The model under review builds one solid part; all positions refer to its coordinate system, in mm. A direction names the side the tool comes from. Coordinates: 2 decimals unless noted, no trailing zeros. Order: outer loops, then holes, each group sorted by start corner. A loop starts at its lowest first (then second) coordinate and runs counter-clockwise, first axis right, second up.
Autodesk Inventor part; units mm, degrees
ref_plane "YZ Plane" through (0, 0, 0) normal (1, 0, 0) x (0, 1, 0)
ref_plane "XZ Plane" through (0, 0, 0) normal (0, 1, 0) x (-1, 0, 0)
ref_plane "XY Plane" through (0, 0, 0) normal (0, 0, 1) x (1, 0, 0)
sketch "Sketch1" plane through (0, 0, 0) normal (0, 1, 0) x (-1, 0, 0)
  circle A0 centre (0, 0) radius 7.5
  dimension "d8" = 15
extrude "Extrusion1" add sketch "Sketch1" along normal blind 53
sketch "Sketch2" plane through (0, 0, 0) normal (0, -1, 0) x (1, 0, 0)
  circle A0 centre (0, 0) radius 1.5
  dimension "d3" = 3
extrude "Extrusion2" add sketch "Sketch2" along normal blind 2
fillet "Fillet1" [suppressed]
fillet "Fillet2" radius 0.4 2 edges at (-1.5, -2, 0) (-1.5, 0, 0)
fillet "Fillet3" radius 1 2 edges at (7.5, 53, 0) (7.5, 0, 0)
properties part number "Battery"
(1) Machinability: for faces 1 (the face through (0, -2, 0)), 2 (the face through (-1, 0, 2)), which of the approach directions +Z, -Z, +X, -X, +Y, -Y give a long, thin tool a straight path to every point of the face, cutting with its end or side? Answer none if there is none.
A:
face 1: +Z, -Z, +X, -X, -Y
face 2: -Y
(2) We need section B-B, the plane z = 0. Write out the cut boundary in (x, y).
A:
outline: (-7.5, 1) arc R1 ccw to (-6.5, 0) - (-1.9, 0) arc R0.4 cw to (-1.5, -0.4) - (-1.5, -1.6) arc R0.4 ccw to (-1.1, -2) - (1.1, -2) arc R0.4 ccw to (1.5, -1.6) - (1.5, -0.4) arc R0.4 cw to (1.9, 0) - (6.5, 0) arc R1 ccw to (7.5, 1) - (7.5, 52) arc R1 ccw to (6.5, 53) - (-6.5, 53) arc R1 ccw to (-7.5, 52) - close
(3) Wall thickness on probe 1 along Y at (x, z) = (0.25, 5.25); probe 2 along Z at (x, y) = (0.25, 42); probe 3 along Z at (x, y) = (2, 40.5): over which ranges is each line inside the solid? List them lowest first.
A:
probe 1: y = 0 to 53
probe 2: z = -7.5 to 7.5
probe 3: z = -7.23 to 7.23
(4) We need section C-C, the plane y = 33. Write out the cut boundary in (x, z), and give its area (3 significant figures).
A:
outline: circle Ø15 at (0, 0)
area: 177 mm2
(5) For pin 1 Ø5 at (x, y) = (3, 44) entering from -Z; pin 2 Ø3 at (x, z) = (-1.5, -3.5) entering from -Y; pin 3 Ø3 at (x, y) = (5, 38) entering from +Z, all flat-tipped, find the tip position at first contact; note any pin that passes through.
A:
pin 1: stops at z = -7.48
pin 2: stops at y = 0
pin 3: stops at z = 6.63
(6) We need section A-A, the plane x = 0. Write out the cut boundary in (y, z), and give its area (3 significant figures).
A:
outline: (-2, -1.1) arc R0.4 ccw to (-1.6, -1.5) - (-0.4, -1.5) arc R0.4 cw to (0, -1.9) - (0, -6.5) arc R1 ccw to (1, -7.5) - (52, -7.5) arc R1 ccw to (53, -6.5) - (53, 6.5) arc R1 ccw to (52, 7.5) - (1, 7.5) arc R1 ccw to (0, 6.5) - (0, 1.9) arc R0.4 cw to (-0.4, 1.5) - (-1.6, 1.5) arc R0.4 ccw to (-2, 1.1) - close
area: 800 mm2
